Model file for the job. Use its own axes, mm. Face numbers are marked on the shaded views. A direction names the side the tool comes from. Round coordinates to 2 decimals unless told otherwise and drop trailing zeros. Loops run counter-clockwise (first coordinate to the right, second up) from the corner with the lowest first, then second, coordinate; pieces in that order, holes last. Notation, with made-up numbers: (52.25, -0.5) -> (84.25, -0.5) arc R29 ccw to (84.25, 37.5) -> close; hole circle Ø8 at (64, -24). An arc over 180 degrees is marked (long way). Use a Markdown table: item, result. Add a question column.
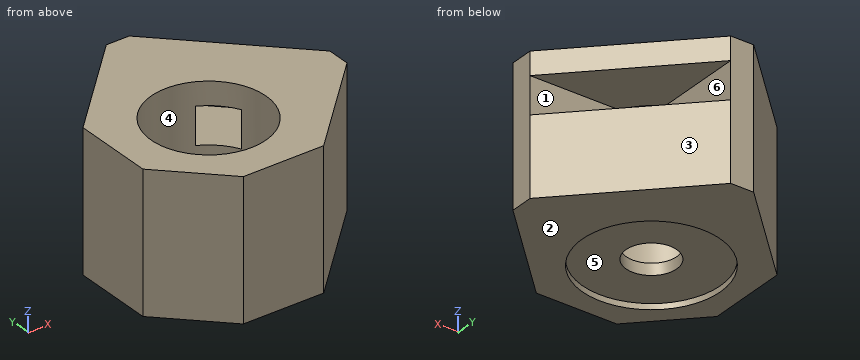
```python
from build123d import *

# Parameters (mm, degrees)
ESQUISSE1_W             = 20
ESQUISSE1_H             = 20
BOSS_EXTRU_1_DEPTH      = 12
CHANFREIN1_SIZE         = 10
ENL_V_START             = -2
ENL_V_MAT_EXTRU_1_DEPTH = 3.2
ESQUISSE3_R             = 2.2
ENL_V_MAT_EXTRU_2_DEPTH = 13
ESQUISSE4_R             = 5
ENL_V_MAT_EXTRU_3_DEPTH = 10.5
CHANFREIN2_SIZE         = 5
CHANFREIN3_SIZE         = 8
SKETCH1_R               = 6
CUT_EXTRUDE1_DEPTH      = 0.5


with BuildPart() as part:
    # Esquisse1 → Boss.-Extru.1 (new body)
    with BuildSketch(Plane.XY):
        with Locations((10, 10)):
            Rectangle(ESQUISSE1_W, ESQUISSE1_H)
    extrude(amount=BOSS_EXTRU_1_DEPTH)

    # Chanfrein1
    chanfrein1_edges = [part.edges().sort_by_distance(p)[0] for p in [
        (20, 20, 6),
    ]]
    chamfer(chanfrein1_edges, length=CHANFREIN1_SIZE)

    # Esquisse2 → Enlèv. mat.-Extru.1 (cut)
    with BuildSketch(Plane.XY.offset(12).offset(ENL_V_START)):
        Polygon((10, 20), (10, 10), (20, 10), align=None)
    extrude(amount=-ENL_V_MAT_EXTRU_1_DEPTH, mode=Mode.SUBTRACT)

    # Esquisse3 → Enlèv. mat.-Extru.2 (cut, through all)
    with BuildSketch(Plane(origin=(0, 0, 0), x_dir=(-1, 0, 0), z_dir=(0, 0, -1))):
        with Locations((-7.8, 7.8)):
            Circle(ESQUISSE3_R)
    extrude(amount=-ENL_V_MAT_EXTRU_2_DEPTH, mode=Mode.SUBTRACT)

    # Esquisse4 → Enlèv. mat.-Extru.3 (cut)
    with BuildSketch(Plane.XY.offset(12)):
        with Locations((7.8, 7.8)):
            Circle(ESQUISSE4_R)
    extrude(amount=-ENL_V_MAT_EXTRU_3_DEPTH, mode=Mode.SUBTRACT)

    # Chanfrein2
    chanfrein2_edges = [part.edges().sort_by_distance(p)[0] for p in [
        (0, 0, 6),
    ]]
    chamfer(chanfrein2_edges, length=CHANFREIN2_SIZE)

    # Chanfrein3
    chanfrein3_edges = [part.edges().sort_by_distance(p)[0] for p in [
        (0, 20, 6),
        (20, 0, 6),
    ]]
    chamfer(chanfrein3_edges, length=CHANFREIN3_SIZE)

    # Sketch1 → Cut-Extrude1 (cut)
    with BuildSketch(Plane(origin=(0, 0, 0), x_dir=(-1, 0, 0), z_dir=(0, 0, -1))):
        with Locations((-7.8, 7.8)):
            Circle(SKETCH1_R)
    extrude(amount=-CUT_EXTRUDE1_DEPTH, mode=Mode.SUBTRACT)


solid = part.part
```
1) Cut at D-D on z = 8.5. Write the cut outline in (x, y), and give its area (3 significant figures).
2) Pin check, flat tips, straight feed: pin 1 Ø3.5 at (x, y) = (9.5, 8.5) entering from -Z; pin 2 Ø1 at (y, z) = (17.5, 8) entering from +X; pin 3 Ø1.5 at (y, z) = (14.5, 8) entering from -X. Stop position of each tip, or through.
3) Cut at B-B on x = 18.25. Write the cut outline in (y, z).
4) Wall check: probe 1 along Z at (x, y) = (10.75, 16.25); probe 2 along Z at (x, y) = (11.25, 12.25); probe 3 along Z at (x, y) = (2.5, 7.25). Give the ranges that are in metal, low to high. Write a range as from..to.
5) Cut at A-A on z = 4.75. Write the cut outline in (x, y), and give its area (3 significant figures).
6) Pull direction Y, two halves, no side cores. Call the marked faces 3, 4, 5 and 6: +Y half, -Y half, draft (parallel to the pull), parting line (faces both ways), or undercut.
7) Tool access for the marked faces 1 and 2: list every direction of +Z, -Z, +X, -X, +Y, -Y with a clear straight run to the whole face (end or side of a thin tool).
8) Cut at C-C on y = 15.75. Write the cut outline in (x, z), and give its area (3 significant figures).
Established:
| question | item | result |
|---|---|---|
| 1 | outline | (0, 5) -> (5, 0) -> (12, 0) -> (20, 8) -> (20, 10) -> (12.29, 10) arc R5 cw (long way) to (10, 12.29) -> (10, 20) -> (8, 20) -> (0, 12) -> close |
| 1 | area | 148 mm^2 |
| 2 | pin 1 | stops at z = 0.5 |
| 2 | pin 2 | stops at x = 10 |
| 2 | pin 3 | stops at x = 1.75 |
| 3 | outline | (6.25, 0) -> (11.75, 0) -> (11.75, 6.8) -> (10, 6.8) -> (10, 10) -> (11.75, 10) -> (11.75, 12) -> (6.25, 12) -> close |
| 4 | probe 1 | z = 0..6.8, 10..12 |
| 4 | probe 2 | z = 0.5..6.8, 10..12 |
| 4 | probe 3 | z = 0.5..12 |
| 5 | outline | (0, 5) -> (5, 0) -> (12, 0) -> (20, 8) -> (20, 10) -> (10, 20) -> (8, 20) -> (0, 12) -> close; hole circle Ø10 at (7.8, 7.8) |
| 5 | area | 195 mm^2 |
| 6 | face 3 | +Y half |
| 6 | face 4 | undercut |
| 6 | face 5 | undercut |
| 6 | face 6 | draft |
| 7 | face 1 | +X, +Y |
| 7 | face 2 | -Z, +X, -X, +Y, -Y |
| 8 | outline | (3.75, 0) -> (14.25, 0) -> (14.25, 6.8) -> (10, 6.8) -> (10, 10) -> (14.25, 10) -> (14.25, 12) -> (3.75, 12) -> close |
| 8 | area | 112 mm^2 |
